Job drawing, mm, ordinate dimensions from the low corner. One solid piece. A direction names the side the tool comes from. Coordinates: 2 decimals unless noted, no trailing zeros. Loops run counter-clockwise (first coordinate to the right, second up) from the corner with the lowest first, then second, coordinate; pieces in that order, holes last. Notation, with made-up numbers: (-27, -9) - (5, -9) arc R26 ccw to (5, 9) - close; hole circle Ø9 at (-20, -19.5). An arc over 180 degrees is marked (long way). Use a Markdown table: item, result. Add a question column.
1) Pull direction X, two halves, no side cores. Call the marked faces 1, 2 and 3: +X half, -X half, draft (parallel to the pull), parting line (faces both ways), or undercut.
2) Band-saw the part on C-C (x = 76.5). Give the cut face in (y, z).
3) Drop flat-ended pins along their axis: P1, Ø8, axis at x = 29.5, z = 20.5, coming from the -Y side; P2, Ø4.5, axis at x = 53.5, z = 12, coming from the -Y side. Give the stop position or say it passes through.
4) Band-saw the part on A-A (x = 51.5). Give the cut face in (y, z), plus the area to 3 significant figures.
5) Band-saw the part on B-B (z = 25.5). Give the cut face in (x, y) (1 decimal).
6) Probe probe 1 along X at (y, z) = (2.1, 8.5) (1 decimal); probe 2 along X at (y, z) = (0.2, 16) (1 decimal); probe 3 along X at (y, z) = (1.25, 27) (1 decimal). List the from-to ranges inside material, lowest first. Write a range as [from, to].
7) Tool access for the marked faces 4 and 5: list every direction of +Z, -Z, +X, -X, +Y, -Y with a clear straight run to the whole face (end or side of a thin tool).
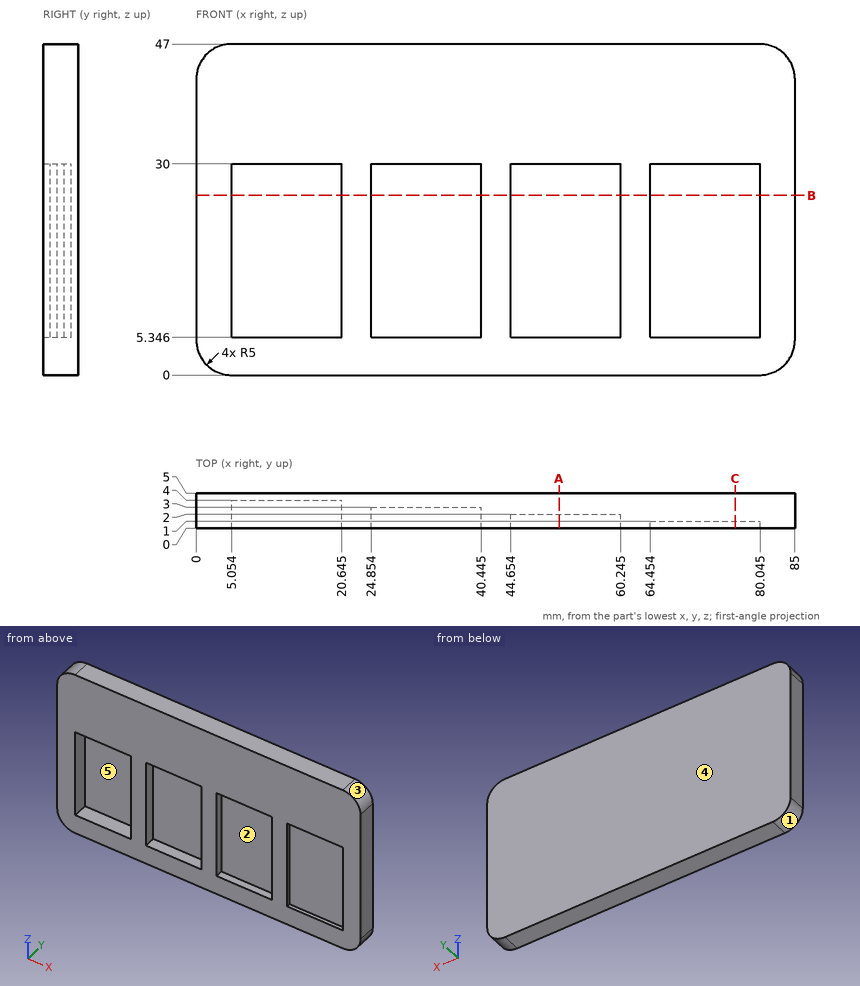
Answer block:
| question | item | result |
|---|---|---|
| 1 | face 1 | -X half |
| 1 | face 2 | undercut |
| 1 | face 3 | +X half |
| 2 | outline | (0, 0) - (5, 0) - (5, 47) - (0, 47) - (0, 30) - (1, 30) - (1, 5.35) - (0, 5.35) - close |
| 3 | P1 | y = 3 |
| 3 | P2 | y = 2 |
| 4 | outline | (0, 0) - (5, 0) - (5, 47) - (0, 47) - (0, 30) - (2, 30) - (2, 5.35) - (0, 5.35) - close |
| 4 | area | 186 mm2 |
| 5 | outline | (0, 0) - (5.1, 0) - (5.1, 4) - (20.6, 4) - (20.6, 0) - (24.9, 0) - (24.9, 3) - (40.4, 3) - (40.4, 0) - (44.7, 0) - (44.7, 2) - (60.2, 2) - (60.2, 0) - (64.5, 0) - (64.5, 1) - (80, 1) - (80, 0) - (85, 0) - (85, 5) - (0, 5) - close |
| 6 | probe 1 | [0, 5.1], [20.6, 24.9], [40.4, 85] |
| 6 | probe 2 | [0, 5.1], [20.6, 24.9], [40.4, 44.7], [60.2, 64.5], [80, 85] |
| 6 | probe 3 | [0, 5.1], [20.6, 24.9], [40.4, 44.7], [60.2, 85] |
| 7 | face 4 | +Z, -Z, +X, -X, +Y |
| 7 | face 5 | -Y |
